The model under review builds one solid part; all positions refer to its coordinate system, in mm. A direction names the side the tool comes from. Round coordinates to 2 decimals unless told otherwise and drop trailing zeros. Order: outer loops, then holes, each group sorted by start corner. A loop starts at its lowest first (then second) coordinate and runs counter-clockwise, first axis right, second up. Notation, with made-up numbers: M -34.5,34 L -24.5,34 A34 cw -24.5,72 Z; hole C 19,36 d10. An arc over 180 degrees is marked long. One line per item, written item: value. Start each with the question number.
from build123d import *

# Parameters (mm, degrees)
F0_W     = 28
F0_H     = 100
F1_DEPTH = 25
F3_D     = 4.5
F3_DEPTH = 8.5
F3_TIP   = 1.3519363928
F4_W     = 28
F4_H     = 8
F5_DEPTH = 100.001


with BuildPart() as f1:
    # F0 (on Front) → F1 (new body)
    with BuildSketch(Plane.XZ):
        with Locations((14, 50)):
            Rectangle(F0_W, F0_H)
        with BuildLine():
            Line((14, 97), (22, 97))
            ThreePointArc((22, 97), (22.7071067812, 96.7071067812), (23, 96))
            Line((23, 96), (23, 9.0192308693))
            Line((23, 9.0192308693), (3, 9.0192308693))
            Line((3, 9.0192308693), (3, 87.5))
            ThreePointArc((3, 87.5), (3.2928932188, 88.2071067812), (4, 88.5))
            Line((4, 88.5), (10, 88.5))
            ThreePointArc((10, 88.5), (12.1213203436, 89.3786796564), (13, 91.5))
            Line((13, 91.5), (13, 96))
            ThreePointArc((13, 96), (13.2928932188, 96.7071067812), (14, 97))
        make_face(mode=Mode.SUBTRACT)
    extrude(amount=F1_DEPTH)

    # F3
    with Locations(Plane.XY.offset(100)):
        with Locations((6.5, -17)):
            Hole(F3_D / 2, depth=F3_DEPTH)
            with Locations((0, 0, -(F3_DEPTH + F3_TIP / 2))):  # 118° drill point
                Cone(0, F3_D / 2, F3_TIP, mode=Mode.SUBTRACT)

    # F4 (on face) → F5 (cut, through all)
    with BuildSketch(Plane.XY.offset(100)):
        with Locations((14, -21)):
            Rectangle(F4_W, F4_H)
    extrude(amount=-F5_DEPTH, mode=Mode.SUBTRACT)


solid = f1.part
Item 1: Machinability: for faces 1 (the cylindrical face through (6.45, -14.75, 95.69)), 2 (the cylindrical face through (12.1, -8.38, 89.36)), 3 (the flat face through (26, -17, 40)), which of the approach directions +Z, -Z, +X, -X, +Y, -Y give a long, thin tool a straight path to every point of the face, cutting with its end or side? Answer none if there is none.
Item 2: The part is to be moulded in two halves that separate along X. For faces 4 (the flat face through (28, -8, 49)), 5 (the flat face through (26, 0, 51)), 6 (the conical face through (6.52, -16.109, 90.683)), 7 (the flat face through (0, -8, 49)), say which applies: pulls with the +X half, pulls with the -X half, needs draft (parallel to the pull), parting line crosses it, or undercut.
Item 3: Consider section A-A, the plane z = 71.5. Give the boundary of the cut face in (x, y), then the cut area to 3 significant figures.
Item 4: Consider section C-C, the plane y = -12.5. Give the boundary of the cut face in (x, z), then the cut area to 3 significant figures.
Item 5: Consider section B-B, the plane x = 6.5. Give the boundary of the cut face in (y, z), then the cut area to 3 significant figures.
Item 6: Wall thickness on L1, parallel to Z at x = 5, y = -15.25; L2, parallel to Z at x = 17.5, y = -6.5; L3, parallel to X at y = -12, z = 54.5: over which ranges is each line inside the solid? List them lowest first.
Computed:
1. face 1: +Z, -Y
1. face 2: +Y, -Y
1. face 3: +Z, -Z, +X, -X, -Y
2. face 4: pulls with the +X half
2. face 5: needs draft
2. face 6: undercut
2. face 7: pulls with the -X half
3. outline: M 0,-17 L 3,-17 L 3,0 L 0,0 Z; M 23,-17 L 28,-17 L 28,0 L 23,0 Z
3. area: 136 mm^2
4. outline: M 0,0 L 28,0 L 28,100 L 0,100 Z; hole M 3,9.02 L 23,9.02 L 23,96 A1 ccw 22,97 L 14,97 A1 ccw 13,96 L 13,91.5 A3 cw 10,88.5 L 4,88.5 A1 ccw 3,87.5 Z
4. area: 1,120 mm^2
5. outline: M -17,0 L 0,0 L 0,9.02 L -17,9.02 Z; M -17,88.5 L 0,88.5 L 0,100 L -14.75,100 L -14.75,91.5 L -17,90.15 Z
5. area: 328 mm^2
6. L1: z = 0 to 9.02, 88.5 to 100
6. L2: z = 0 to 9.02, 97 to 100
6. L3: x = 0 to 3, 23 to 28
